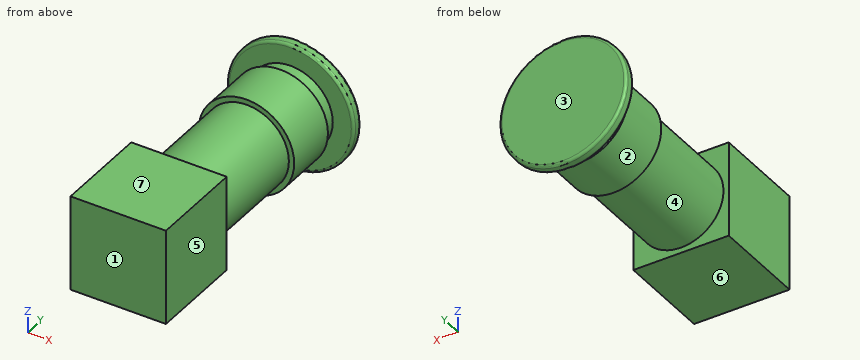
```python
from build123d import *

# Parameters (mm, degrees)
ESQUISSE1_W        = 18
ESQUISSE1_H        = 18
BOSS_EXTRU_1_DEPTH = 18
ESQUISSE2_R        = 8
BOSS_EXTRU_2_DEPTH = 20
ESQUISSE3_R        = 9
BOSS_EXTRU_3_DEPTH = 10
ESQUISSE4_R        = 8
BOSS_EXTRU_4_DEPTH = 3
ESQUISSE5_R        = 12
BOSS_EXTRU_5_DEPTH = 2
CONG_1_R           = 0.5
CONG_2_R           = 0.5


with BuildPart() as part:
    # Esquisse1 → Boss.-Extru.1 (new body)
    with BuildSketch(Plane(origin=(0, 0, 0), x_dir=(1, 0, 0), z_dir=(0, 1, 0))):
        Rectangle(ESQUISSE1_W, ESQUISSE1_H)
    extrude(amount=BOSS_EXTRU_1_DEPTH)

    # Esquisse2 → Boss.-Extru.2 (add)
    with BuildSketch(Plane(origin=(0, 18, 0), x_dir=(1, 0, 0), z_dir=(0, 1, 0))):
        Circle(ESQUISSE2_R)
    extrude(amount=BOSS_EXTRU_2_DEPTH)

    # Esquisse3 → Boss.-Extru.3 (add)
    with BuildSketch(Plane(origin=(0, 38, 0), x_dir=(1, 0, 0), z_dir=(0, 1, 0))):
        Circle(ESQUISSE3_R)
    extrude(amount=BOSS_EXTRU_3_DEPTH)

    # Esquisse4 → Boss.-Extru.4 (add)
    with BuildSketch(Plane(origin=(0, 48, 0), x_dir=(1, 0, 0), z_dir=(0, 1, 0))):
        Circle(ESQUISSE4_R)
    extrude(amount=BOSS_EXTRU_4_DEPTH)

    # Esquisse5 → Boss.-Extru.5 (add)
    with BuildSketch(Plane(origin=(0, 51, 0), x_dir=(1, 0, 0), z_dir=(0, 1, 0))):
        Circle(ESQUISSE5_R)
    extrude(amount=BOSS_EXTRU_5_DEPTH)

    # Congé1
    cong_1_edges = [part.edges().sort_by_distance(p)[0] for p in [
        (-12, 53, 0),
    ]]
    fillet(cong_1_edges, radius=CONG_1_R)

    # Congé2
    cong_2_edges = [part.edges().sort_by_distance(p)[0] for p in [
        (-12, 51, 0),
    ]]
    fillet(cong_2_edges, radius=CONG_2_R)


solid = part.part
```
Geometry check sheet. Reference: the model listing, model coordinates, mm. Face numbers are marked on the shaded views. A direction names the side the tool comes from. Coordinates: 2 decimals unless noted, no trailing zeros. Order: outer loops, then holes, each group sorted by start corner. A loop starts at its lowest first (then second) coordinate and runs counter-clockwise, first axis right, second up. Notation, with made-up numbers: (-2.5, 7.5) - (5.5, 7.5) arc R7 ccw to (5.5, 20.5) - close; hole circle Ø8 at (-25.75, -32.5). An arc over 180 degrees is marked (long way). Answer in a Markdown table with one row per item. Add a question column.
1. Access from +Z, -Z, +X, -X, +Y, -Y to the whole of each face (thin tool, end or side, straight path). Record for the marked faces 4, 5, 6 and 7.
2. Section check B-B (x = 0). Enter the section's corners in (y, z).
3. Section check D-D (y = 46). Enter the section's corners in (x, z), plus the area to 3 significant figures.
4. Draft check along Y on the marked faces 1, 2 and 3. Enter one of: +Y half, -Y half, draft (parallel to the pull), parting line (faces both ways), or undercut.
5. Section check A-A (z = 0). Enter the section's corners in (x, y).
6. Gauge pin test, flat ends, axial feed: pin 1 Ø5 at (y, z) = (27.5, 3.5) entering from -X; pin 2 Ø12 at (y, z) = (7, -1.5) entering from +X; pin 3 Ø5 at (y, z) = (22, -1) entering from -X. Record the tip position at first contact, or that the pin passes through.
7. Section check C-C (y = 5.5). Enter the section's corners in (x, z), plus the area to 3 significant figures.
8. Material ranges on L1, parallel to Y at x = 8, z = 2; L2, parallel to Y at x = -5.5, z = 8.25; L3, parallel to Z at x = -1, y = 12, recorded low to high. Write a range as [from, to].
Data:
| question | item | result |
|---|---|---|
| 1 | face 4 | none |
| 1 | face 5 | +Z, -Z, +X, -Y |
| 1 | face 6 | -Z, +X, -X, -Y |
| 1 | face 7 | +Z, +X, -X, -Y |
| 2 | outline | (0, -9) - (18, -9) - (18, -8) - (38, -8) - (38, -9) - (48, -9) - (48, -8) - (51, -8) - (51, -11.5) arc R0.5 ccw to (51.5, -12) - (52.5, -12) arc R0.5 ccw to (53, -11.5) - (53, 11.5) arc R0.5 ccw to (52.5, 12) - (51.5, 12) arc R0.5 ccw to (51, 11.5) - (51, 8) - (48, 8) - (48, 9) - (38, 9) - (38, 8) - (18, 8) - (18, 9) - (0, 9) - close |
| 3 | outline | circle Ø18 at (0, 0) |
| 3 | area | 254 mm² |
| 4 | face 1 | -Y half |
| 4 | face 2 | undercut |
| 4 | face 3 | +Y half |
| 5 | outline | (-12, 51.5) arc R0.5 ccw to (-11.5, 51) - (-8, 51) - (-8, 48) - (-9, 48) - (-9, 38) - (-8, 38) - (-8, 18) - (-9, 18) - (-9, 0) - (9, 0) - (9, 18) - (8, 18) - (8, 38) - (9, 38) - (9, 48) - (8, 48) - (8, 51) - (11.5, 51) arc R0.5 ccw to (12, 51.5) - (12, 52.5) arc R0.5 ccw to (11.5, 53) - (-11.5, 53) arc R0.5 ccw to (-12, 52.5) - close |
| 6 | pin 1 | stops at x = -7.94 |
| 6 | pin 2 | stops at x = 9 |
| 6 | pin 3 | stops at x = -8 |
| 7 | outline | (-9, -9) - (9, -9) - (9, 9) - (-9, 9) - close |
| 7 | area | 324 mm² |
| 8 | L1 | y = [0, 18], [38, 48], [51, 53] |
| 8 | L2 | y = [0, 18], [51, 53] |
| 8 | L3 | z = [-9, 9] |
